```python
from build123d import *

# Parameters (mm, degrees)
BOSS_EXTRUDE1_DEPTH = 23.4
FILLET1_R           = 4
FILLET3_R           = 2
FILLET4_R           = 4
FILLET5_R           = 5
BOSS_EXTRUDE2_DEPTH = 24.5
BOSS_EXTRUDE3_START = 8
SKETCH3_R           = 0.75
BOSS_EXTRUDE3_DEPTH = 8


with BuildPart() as part:
    # Sketch1 → Boss-Extrude1 (new body)
    with BuildSketch(Plane(origin=(0, 0, 0), x_dir=(1, 0, 0), z_dir=(0, 1, 0))):
        with BuildLine():
            Line((0, 0), (30, 0))
            Line((30, 0), (30, 5.1))
            Line((30, 5.1), (36.395958363, 2.511232605))
            ThreePointArc((36.395958363, 2.511232605), (37.463728778, 1.925417586), (38.366240646, 1.107624688))
            Line((38.366240646, 1.107624688), (42.902523658, -4.091619145))
            ThreePointArc((42.902523658, -4.091619145), (43.590417547, -5.096663868), (44.026071732, -6.233993339))
            Line((44.026071732, -6.233993339), (45.723869414, -12.921854211))
            ThreePointArc((45.723869414, -12.921854211), (45.883457457, -14.129266548), (45.7582513, -15.340726954))
            Line((45.7582513, -15.340726954), (44.251223786, -22.074141249))
            ThreePointArc((44.251223786, -22.074141249), (43.848071102, -23.223393532), (43.189020782, -24.247583736))
            Line((43.189020782, -24.247583736), (38.802344779, -29.573658617))
            ThreePointArc((38.802344779, -29.573658617), (37.883123065, -30.501625481), (36.810104599, -31.246422387))
            Line((36.810104599, -31.246422387), (28.716751538, -35.827648886))
            ThreePointArc((28.716751538, -35.827648886), (23.339920043, -38.206219709), (17.601311476, -39.485394366))
            ThreePointArc((17.601311476, -39.485394366), (9.20703571, -39.890619172), (0.842295428, -39.078712278))
            Line((0.842295428, -39.078712278), (0.505393215, -41.050132299))
            ThreePointArc((0.505393215, -41.050132299), (9.158517062, -41.89003057), (17.842194661, -41.470835196))
            ThreePointArc((17.842194661, -41.470835196), (22.730520814, -40.484713163), (27.40515094, -38.748048996))
            Line((27.40515094, -38.748048996), (30.194566538, -38.438407937))
            Line((30.194566538, -38.438407937), (38.287919599, -33.857181439))
            ThreePointArc((38.287919599, -33.857181439), (39.812213821, -32.79914781), (41.11802951, -31.480909053))
            Line((41.11802951, -31.480909053), (45.504705513, -26.154834172))
            ThreePointArc((45.504705513, -26.154834172), (46.543404661, -24.540654707), (47.178795219, -22.729370603))
            Line((47.178795219, -22.729370603), (48.685822733, -15.995956308))
            ThreePointArc((48.685822733, -15.995956308), (48.883154446, -14.086628819), (48.63163501, -12.183681305))
            Line((48.63163501, -12.183681305), (46.933837328, -5.495820434))
            ThreePointArc((46.933837328, -5.495820434), (46.247222637, -3.703327329), (45.163064455, -2.119322184))
            Line((45.163064455, -2.119322184), (40.626781443, 3.07992165))
            ThreePointArc((40.626781443, 3.07992165), (39.204373652, 4.368807735), (37.521509404, 5.292084068))
            Line((37.521509404, 5.292084068), (31.475993381, 7.739009747))
            ThreePointArc((31.475993381, 7.739009747), (27.794609995, 8.831354958), (23.972319774, 9.2))
            Line((23.972319774, 9.2), (0, 9.2))
            ThreePointArc((0, 9.2), (-2.867725571, 8.498272017), (-5.087407296, 6.551663389))
            Line((-5.087407296, 6.551663389), (-15.452573661, -8.251328295))
            Line((-15.452573661, -8.251328295), (-13.40469355, -9.685269386))
            ThreePointArc((-13.40469355, -9.685269386), (-14.36147987, -12.463471121), (-13.70098006, -15.326613615))
            Line((-13.70098006, -15.326613615), (-15.013073156, -16.053532941))
            Line((-15.013073156, -16.053532941), (-4.642357438, -34.772727782))
            Line((-4.642357438, -34.772727782), (-2.892899976, -33.803502014))
            ThreePointArc((-2.892899976, -33.803502014), (-0.356026186, -36.605109272), (3.160716272, -37.98975881))
            ThreePointArc((3.160716272, -37.98975881), (18.191080341, -37.623613679), (32.244088475, -32.279563836))
            Line((32.244088475, -32.279563836), (31.228009552, -30.556896247))
            ThreePointArc((31.228009552, -30.556896247), (17.805759331, -35.661082732), (3.450021006, -36.010793734))
            ThreePointArc((3.450021006, -36.010793734), (0.781528732, -34.960126351), (-1.143442514, -32.834276246))
            Line((-1.143442514, -32.834276246), (-11.514158233, -14.115081405))
            ThreePointArc((-11.514158233, -14.115081405), (-11.864920764, -12.594591782), (-11.35681344, -11.119210477))
            Line((-11.35681344, -11.119210477), (0, 5.1))
            Line((0, 5.1), (0, 0))
        make_face()
    extrude(amount=BOSS_EXTRUDE1_DEPTH)

    # Fillet1
    # the kernel refuses this fillet: 4 mm, written as the material it adds along each edge
    with BuildSketch(Plane(origin=(30, 0, -5.1), x_dir=(0, 0, 1), z_dir=(0, 1, 0))) as fillet1_piece_1:
        with BuildLine():
            CenterArc((5.901400798, 3.918897391), FILLET1_R, 157.964334143, 100.478227364)
            Line((2.193598849, 5.419632112), (2.11944281, 5.449646807))
            Line((2.11944281, 5.449646807), (-0.074156039, 0.030014694))
            Line((-0.074156039, 0.030014694), (0, -0.08))
            ThreePointArc((0, -0.08), (2.55, -0.08), (5.083971984, -0.078377948))
            Line((5.083971984, -0.078377948), (5.1, 0))
        make_face()
    extrude(amount=23.4)

    # Fillet3
    # the kernel refuses this fillet: 2 mm, written as the material it adds along each edge
    with BuildSketch(Plane(origin=(0, 0, -5.1), x_dir=(0, 0, 1), z_dir=(0, 1, 0))) as fillet3_piece_1:
        with BuildLine():
            CenterArc((6.021753736, -1.774928182), FILLET3_R, 117.443704679, 117.556295321)
            Line((4.874600863, -3.41323227), (4.851657806, -3.445998352))
            Line((4.851657806, -3.445998352), (-0.022943057, -0.032766082))
            Line((-0.022943057, -0.032766082), (0, 0.04))
            ThreePointArc((0, 0.04), (2.55, 0.04), (5.081564925, 0.035498564))
            Line((5.081564925, 0.035498564), (5.1, 0))
        make_face()
    extrude(amount=23.4)

    # Fillet4
    fillet4_edges = [part.edges().sort_by_distance(p)[0] for p in [
        (0, 11.7, 0),
    ]]
    fillet(fillet4_edges, radius=FILLET4_R)

    # Fillet5
    fillet5_edges = [part.edges().sort_by_distance(p)[0] for p in [
        (30, 11.7, 0),
    ]]
    fillet(fillet5_edges, radius=FILLET5_R)

    # Sketch2 → Boss-Extrude2 (add)
    with BuildSketch(Plane(origin=(0, 23.4, 0), x_dir=(1, 0, 0), z_dir=(0, 1, 0))):
        with BuildLine():
            Line((-4.642357438, -34.772727782), (-2.892899976, -33.803502014))
            Line((-2.892899976, -33.803502014), (-1.143442514, -32.834276246))
            Line((-1.143442514, -32.834276246), (-11.514158233, -14.115081405))
            ThreePointArc((-11.514158233, -14.115081405), (-11.864920764, -12.594591782), (-11.35681344, -11.119210477))
            Line((-11.35681344, -11.119210477), (-3.41323227, 0.225399137))
            ThreePointArc((-3.41323227, 0.225399137), (-2.124184908, 1.047515098), (-0.631039096, 0.718830843))
            ThreePointArc((-0.631039096, 0.718830843), (0.457713769, 0.183936804), (1.656739075, 0))
            Line((1.656739075, 0), (27.038218008, 0))
            ThreePointArc((27.038218008, 0), (29.145941635, 0.465961942), (30.860817665, 1.776999556))
            ThreePointArc((30.860817665, 1.776999556), (32.957014936, 3.081224878), (35.419632112, 2.906401151))
            Line((35.419632112, 2.906401151), (35.419632112, 5.599970739))
            ThreePointArc((35.419632112, 5.599970739), (33.507981211, 6.780419817), (31.475993381, 7.739009747))
            ThreePointArc((31.475993381, 7.739009747), (27.794609995, 8.831354958), (23.972319774, 9.2))
            Line((23.972319774, 9.2), (0, 9.2))
            ThreePointArc((0, 9.2), (-2.867725571, 8.498272017), (-5.087407296, 6.551663389))
            Line((-5.087407296, 6.551663389), (-15.452573661, -8.251328295))
            Line((-15.452573661, -8.251328295), (-13.40469355, -9.685269386))
            ThreePointArc((-13.40469355, -9.685269386), (-14.36147987, -12.463471121), (-13.70098006, -15.326613615))
            Line((-13.70098006, -15.326613615), (-15.013073156, -16.053532941))
            Line((-15.013073156, -16.053532941), (-4.642357438, -34.772727782))
        make_face()
    extrude(amount=BOSS_EXTRUDE2_DEPTH)

    # Sketch3 → Boss-Extrude3 (add)
    with BuildSketch(Plane.XZ.offset(BOSS_EXTRUDE3_START)):
        with BuildLine():
            Line((27.038218008, 0), (1.656739075, 0))
            ThreePointArc((1.656739075, 0), (0.457713769, -0.183936804), (-0.631039096, -0.718830843))
            ThreePointArc((-0.631039096, -0.718830843), (-2.124184908, -1.047515098), (-3.41323227, -0.225399137))
            Line((-3.41323227, -0.225399137), (-11.35681344, 11.119210477))
            ThreePointArc((-11.35681344, 11.119210477), (-11.864920764, 12.594591782), (-11.514158233, 14.115081405))
            Line((-11.514158233, 14.115081405), (-1.143442514, 32.834276246))
            ThreePointArc((-1.143442514, 32.834276246), (0.781528732, 34.960126351), (3.450021006, 36.010793734))
            ThreePointArc((3.450021006, 36.010793734), (17.805759331, 35.661082732), (31.228009552, 30.556896247))
            Line((31.228009552, 30.556896247), (32.244088475, 32.279563836))
            ThreePointArc((32.244088475, 32.279563836), (18.191080341, 37.623613679), (3.160716272, 37.98975881))
            ThreePointArc((3.160716272, 37.98975881), (-0.356026186, 36.605109272), (-2.892899976, 33.803502014))
            Line((-2.892899976, 33.803502014), (-4.642357438, 34.772727782))
            Line((-4.642357438, 34.772727782), (-15.013073156, 16.053532941))
            Line((-15.013073156, 16.053532941), (-13.70098006, 15.326613615))
            ThreePointArc((-13.70098006, 15.326613615), (-14.36147987, 12.463471121), (-13.40469355, 9.685269386))
            Line((-13.40469355, 9.685269386), (-15.452573661, 8.251328295))
            Line((-15.452573661, 8.251328295), (-5.087407296, -6.551663389))
            ThreePointArc((-5.087407296, -6.551663389), (-2.867725571, -8.498272017), (0, -9.2))
            Line((0, -9.2), (23.972319774, -9.2))
            ThreePointArc((23.972319774, -9.2), (27.794609995, -8.831354958), (31.475993381, -7.739009747))
            Line((31.475993381, -7.739009747), (37.521509404, -5.292084068))
            ThreePointArc((37.521509404, -5.292084068), (39.204373652, -4.368807735), (40.626781443, -3.07992165))
            Line((40.626781443, -3.07992165), (45.163064455, 2.119322184))
            ThreePointArc((45.163064455, 2.119322184), (46.247222637, 3.703327329), (46.933837328, 5.495820434))
            Line((46.933837328, 5.495820434), (48.63163501, 12.183681305))
            ThreePointArc((48.63163501, 12.183681305), (48.883154446, 14.086628819), (48.685822733, 15.995956308))
            Line((48.685822733, 15.995956308), (47.178795219, 22.729370603))
            ThreePointArc((47.178795219, 22.729370603), (46.543404661, 24.540654707), (45.504705513, 26.154834172))
            Line((45.504705513, 26.154834172), (41.11802951, 31.480909053))
            ThreePointArc((41.11802951, 31.480909053), (39.812213821, 32.79914781), (38.287919599, 33.857181439))
            Line((38.287919599, 33.857181439), (30.194566538, 38.438407937))
            Line((30.194566538, 38.438407937), (27.40515094, 38.748048996))
            ThreePointArc((27.40515094, 38.748048996), (22.730520814, 40.484713163), (17.842194661, 41.470835196))
            ThreePointArc((17.842194661, 41.470835196), (9.158517062, 41.89003057), (0.505393215, 41.050132299))
            Line((0.505393215, 41.050132299), (0.842295428, 39.078712278))
            ThreePointArc((0.842295428, 39.078712278), (9.20703571, 39.890619172), (17.601311476, 39.485394366))
            ThreePointArc((17.601311476, 39.485394366), (23.339920043, 38.206219709), (28.716751538, 35.827648886))
            Line((28.716751538, 35.827648886), (36.810104599, 31.246422387))
            ThreePointArc((36.810104599, 31.246422387), (37.883123065, 30.501625481), (38.802344779, 29.573658617))
            Line((38.802344779, 29.573658617), (43.189020782, 24.247583736))
            ThreePointArc((43.189020782, 24.247583736), (43.848071102, 23.223393532), (44.251223786, 22.074141249))
            Line((44.251223786, 22.074141249), (45.7582513, 15.340726954))
            ThreePointArc((45.7582513, 15.340726954), (45.883457457, 14.129266548), (45.723869414, 12.921854211))
            Line((45.723869414, 12.921854211), (44.026071732, 6.233993339))
            ThreePointArc((44.026071732, 6.233993339), (43.590417547, 5.096663868), (42.902523658, 4.091619145))
            Line((42.902523658, 4.091619145), (38.366240646, -1.107624688))
            ThreePointArc((38.366240646, -1.107624688), (37.463728778, -1.925417586), (36.395958363, -2.511232605))
            Line((36.395958363, -2.511232605), (35.419632112, -2.906401151))
            ThreePointArc((35.419632112, -2.906401151), (32.957014936, -3.081224878), (30.860817665, -1.776999556))
            ThreePointArc((30.860817665, -1.776999556), (29.145941635, -0.465961942), (27.038218008, 0))
        make_face()
        with Locations(Location((-4.310418078, 30.709245073, 0), (0, 0, 270))):
            Circle(SKETCH3_R, mode=Mode.SUBTRACT)
        with Locations(Location((32.111644804, 35.612363227, 0), (0, 0, 270))):
            Circle(SKETCH3_R, mode=Mode.SUBTRACT)
        with Locations(Location((14.004070921, -5.292084068, 0), (0, 0, 270))):
            Circle(SKETCH3_R, mode=Mode.SUBTRACT)
    extrude(amount=-BOSS_EXTRUDE3_DEPTH)


solid = part.part
```
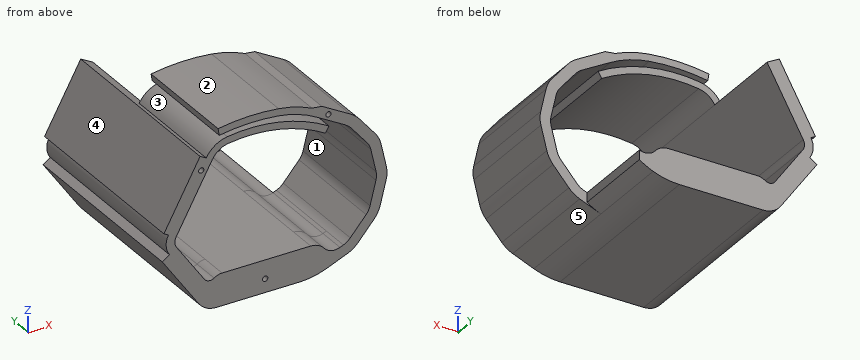
Geometry check sheet. Reference: the model listing, model coordinates, mm. Face numbers are marked on the shaded views. A direction names the side the tool comes from. Give positions to 0.01 mm unless a question says otherwise; leave off trailing zeros. Order: outer loops, then holes, each group sorted by start corner. A loop starts at its lowest first (then second) coordinate and runs counter-clockwise, first axis right, second up. Notation, with made-up numbers: (8, 76.25) -> (41, 76.25) arc R4 cw to (41, 81.25) -> close; hole circle Ø1 at (86, 37.25). An arc over 180 degrees is marked (long way). Write each question's results on one line, items separated by ' | '. Start each with the question number.
(1) Gauge pin test, flat ends, axial feed: P1, Ø2.5, axis at x = 9, z = 36, coming from the +Y side; P2, Ø1, axis at x = 11.5, y = 10.5, coming from the +Z side; P3, Ø6, axis at y = 36, z = -3.5, coming from the -X side. Record the tip position at first contact, or that the pin passes through.
(2) Sectioned sample at B-B (z = 28). Enter the section's corners in (x, y), plus the area to 3 significant figures.
(3) Sectioned sample at C-C (x = 42). Enter the section's corners in (y, z).
(4) Sectioned sample at D-D (y = 43). Enter the section's corners in (x, z), plus the area to 3 significant figures.
(5) Scan lines: line 1 (Z direction, x = 12, y = 17); line 2 (X direction, y = 10, z = 32); line 3 (Z direction, x = 31.5, y = 18.5). Record each from-to range of solid material in increasing order.
(6) Mould release check, pull along Z, two halves, no side actions. Record for the marked faces 3, 4 and 5: pulls with the +Z half, pulls with the -Z half, needs draft (parallel to the pull), parting line crosses it, or undercut.
(7) Access from +Z, -Z, +X, -X, +Y, -Y to the whole of each face (thin tool, end or side, straight path). Record for the marked faces 1 and 2.
(8) Sectioned sample at A-A (x = 25.5). Enter the section's corners in (y, z).
Answer below:
1) P1: y = 23.4 | P2: z = 41.91 | P3: x = -9.32
2) outline: (-8.39, -8) -> (-3.82, -8) -> (-3.82, 47.9) -> (-8.39, 47.9) -> close; (40.1, -8) -> (43.98, -8) -> (43.98, 23.4) -> (40.1, 23.4) -> close | area: 378 mm2
3) outline: (-8, -1.51) -> (23.4, -1.51) -> (23.4, 3.06) -> (-8, 3.06) -> close; (-8, 25.69) -> (23.4, 25.69) -> (23.4, 30.41) -> (-8, 30.41) -> close
4) outline: (-15.45, 8.25) -> (-5.09, -6.55) arc R6.21 ccw to (0, -9.2) -> (23.97, -9.2) arc R20 ccw to (35.42, -5.6) -> (35.42, -2.91) arc R4 cw to (30.86, -1.78) arc R5 ccw to (27.04, 0) -> (1.66, 0) arc R4 ccw to (-0.63, -0.72) arc R2 cw to (-3.41, -0.23) -> (-11.36, 11.12) arc R2.83 cw to (-11.51, 14.12) -> (-1.14, 32.83) -> (-4.64, 34.77) -> (-15.01, 16.05) -> (-13.7, 15.33) arc R5.33 ccw to (-13.4, 9.69) -> close | area: 508 mm2
5) line 1: -9.2 to 0, 36.39 to 38.39, 39.89 to 41.89 | line 2: -6.18 to -1.61, 28.57 to 32.08, 35.48 to 40.66 | line 3: -7.73 to -2.38, 31.02 to 32.71, 34.25 to 37.7
6) face 3: undercut | face 4: pulls with the +Z half | face 5: pulls with the -Z half
7) face 1: +Y, -Y | face 2: +Z, +Y, -Y
8) outline: (-8, -9.14) -> (47.9, -9.14) -> (47.9, 0) -> (-8, 0) -> close; (-8, 33.38) -> (23.4, 33.38) -> (23.4, 35.53) -> (-8, 35.53) -> close; (-8, 37.4) -> (23.4, 37.4) -> (23.4, 39.56) -> (-8, 39.56) -> close
